from build123d import *

# Parameters (mm, degrees)
BOSS_EXTRU_1_DEPTH                                 = 8
ESQUISSE3_R                                        = 1.5
ESQUISSE3_R_2                                      = 5
ENL_V_MAT_EXTRU_1_DEPTH                            = 9
ESQUISSE4_R                                        = 10
ENL_V_MAT_EXTRU_2_DEPTH                            = 9
CHAMBRAGE_POUR_VIS_T_TE_CYLINDRIQUE_CO_D           = 3
CHAMBRAGE_POUR_VIS_T_TE_CYLINDRIQUE_CO_CBORE_D     = 5.5
CHAMBRAGE_POUR_VIS_T_TE_CYLINDRIQUE_CO_CBORE_DEPTH = 2


with BuildPart() as part:
    # Esquisse1 → Boss.-Extru.1 (new body)
    with BuildSketch(Plane.XY):
        with BuildLine():
            Line((938.5, 261), (-193, 261))
            ThreePointArc((-193, 261), (-235.426406871, 243.426406871), (-253, 201))
            Line((-253, 201), (-253, 162))
            Line((-253, 162), (913.5, 162))
            ThreePointArc((913.5, 162), (931.17766953, 169.32233047), (938.5, 187))
            Line((938.5, 187), (938.5, 261))
        make_face()
    extrude(amount=BOSS_EXTRU_1_DEPTH)

    # Esquisse3 → Enlèv. mat.-Extru.1 (cut, through all)
    with BuildSketch(Plane.XY.offset(8)):
        with Locations((-211, 198)):
            Circle(ESQUISSE3_R)
        with Locations((-211, 209)):
            Circle(ESQUISSE3_R_2)
        with Locations((-211, 224)):
            Circle(ESQUISSE3_R_2)
        with Locations((-211, 235)):
            Circle(ESQUISSE3_R)
        with Locations((-196, 209)):
            Circle(ESQUISSE3_R_2)
        with Locations((-196, 198)):
            Circle(ESQUISSE3_R)
        with Locations((-196, 224)):
            Circle(ESQUISSE3_R_2)
        with Locations((-196, 235)):
            Circle(ESQUISSE3_R)
        with Locations((-181, 209)):
            Circle(ESQUISSE3_R_2)
        with Locations((-181, 198)):
            Circle(ESQUISSE3_R)
        with Locations((-181, 224)):
            Circle(ESQUISSE3_R_2)
        with Locations((-181, 235)):
            Circle(ESQUISSE3_R)
        with Locations((-166, 209)):
            Circle(ESQUISSE3_R_2)
        with Locations((-166, 198)):
            Circle(ESQUISSE3_R)
        with Locations((-166, 224)):
            Circle(ESQUISSE3_R_2)
        with Locations((-166, 235)):
            Circle(ESQUISSE3_R)
        with Locations((-151, 209)):
            Circle(ESQUISSE3_R_2)
        with Locations((-151, 198)):
            Circle(ESQUISSE3_R)
        with Locations((-151, 224)):
            Circle(ESQUISSE3_R_2)
        with Locations((-151, 235)):
            Circle(ESQUISSE3_R)
        with Locations((-136, 209)):
            Circle(ESQUISSE3_R_2)
        with Locations((-136, 198)):
            Circle(ESQUISSE3_R)
        with Locations((-136, 224)):
            Circle(ESQUISSE3_R_2)
        with Locations((-136, 235)):
            Circle(ESQUISSE3_R)
        with Locations((-121, 209)):
            Circle(ESQUISSE3_R_2)
        with Locations((-121, 198)):
            Circle(ESQUISSE3_R)
        with Locations((-121, 224)):
            Circle(ESQUISSE3_R_2)
        with Locations((-121, 235)):
            Circle(ESQUISSE3_R)
        with Locations((-106, 209)):
            Circle(ESQUISSE3_R_2)
        with Locations((-106, 198)):
            Circle(ESQUISSE3_R)
        with Locations((-106, 224)):
            Circle(ESQUISSE3_R_2)
        with Locations((-106, 235)):
            Circle(ESQUISSE3_R)
    extrude(amount=-ENL_V_MAT_EXTRU_1_DEPTH, mode=Mode.SUBTRACT)

    # Esquisse4 → Enlèv. mat.-Extru.2 (cut, through all)
    with BuildSketch(Plane.XY.offset(8)):
        with Locations((-30, 224)):
            Circle(ESQUISSE4_R)
        with Locations((210, 224)):
            Circle(ESQUISSE4_R)
        with Locations((450, 224)):
            Circle(ESQUISSE4_R)
        with Locations((690, 224)):
            Circle(ESQUISSE4_R)
    extrude(amount=-ENL_V_MAT_EXTRU_2_DEPTH, mode=Mode.SUBTRACT)

    # Chambrage pour vis à tête cylindrique courte six pans creux M31 (through all)
    with Locations(Plane.XY.offset(8)):
        with Locations((-54, 188), (90, 188), (330, 188), (570, 188), (810, 188), (912.5, 188), (912.5, 251), (810, 251), (570, 251), (330, 251), (90, 251), (-243, 174), (-182.768699819, 251)):
            CounterBoreHole(CHAMBRAGE_POUR_VIS_T_TE_CYLINDRIQUE_CO_D / 2, CHAMBRAGE_POUR_VIS_T_TE_CYLINDRIQUE_CO_CBORE_D / 2, CHAMBRAGE_POUR_VIS_T_TE_CYLINDRIQUE_CO_CBORE_DEPTH)


solid = part.part
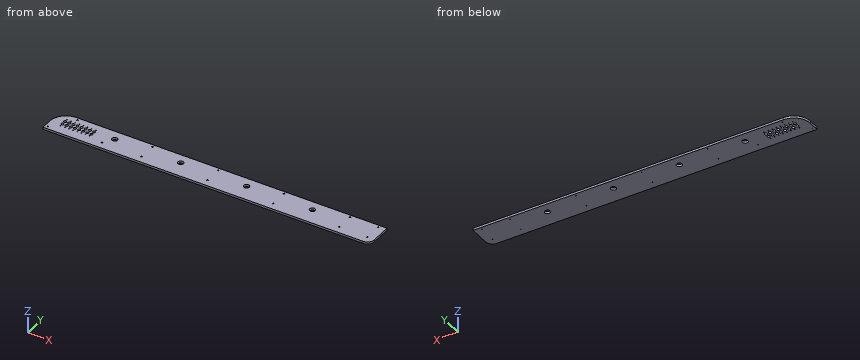
Design review of the part built by this model. Coordinates are the model's own, in mm. Give positions to 0.01 mm unless a question says otherwise; leave off trailing zeros. Order: outer loops, then holes, each group sorted by start corner. A loop starts at its lowest first (then second) coordinate and runs counter-clockwise, first axis right, second up. Notation, with made-up numbers: (64.5, 30.25) - (77.5, 30.25) arc R19 cw to (77.5, 36.25) - close; hole circle Ø5 at (67, 71). An arc over 180 degrees is marked (long way). Write item = value, one per line. Start each with the question number.
Q1. We need section B-B on z = 2.5. State how many separate pieces and enclosed holes the cut face has, plus the area to 3 significant figures.
Q2. We need section A-A on x = -30. State the section outline as (y, z) points, plus the area to 3 significant figures.
Q3. To check wall thickness, follow L1, parallel to Y at x = -181, z = 3.5; L2, parallel to Y at x = 810, z = 7; L3, parallel to Y at x = -28, z = 6.5. State the ranges of each line that lie inside material, in increasing order. Write a range as from..to.
Q4. Clearance check with flat-ended pins moving along their axes: pin 1 Ø1 at (y, z) = (218, 3) entering from -X; pin 2 Ø5 at (x, y) = (330, 251) entering from +Z. State where each tip first meets the part, or that it passes through.
Working result:
q1.separate_pieces = 1
q1.enclosed_holes = 49
q1.area = 114,000 mm²
q2.outline = (162, 0) - (214, 0) - (214, 8) - (162, 8) - close; (234, 0) - (261, 0) - (261, 8) - (234, 8) - close
q2.area = 632 mm²
q3.L1 = 162..196.5, 199.5..204, 214..219, 229..233.5, 236.5..261
q3.L2 = 162..185.25, 190.75..248.25, 253.75..261
q3.L3 = 162..214.2, 233.8..261
q4.pin_1 = -250.69
q4.pin_2 = 6
